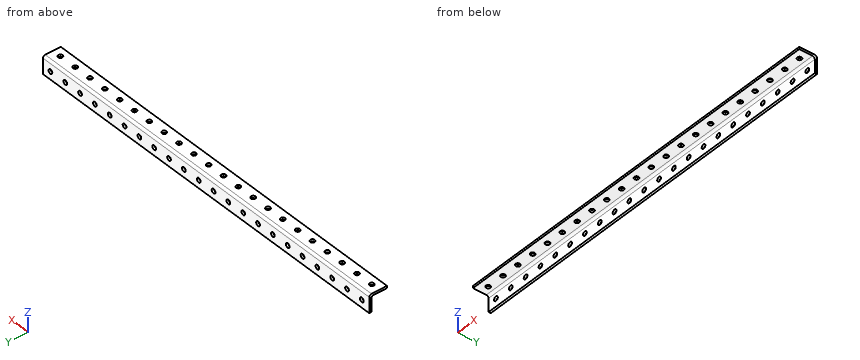
Autodesk Inventor part; units mm, degrees
ref_plane "YZ Plane" through (0, 0, 0) normal (1, 0, 0) x (0, 1, 0)
ref_plane "XZ Plane" through (0, 0, 0) normal (0, 1, 0) x (-1, 0, 0)
ref_plane "XY Plane" through (0, 0, 0) normal (0, 0, 1) x (1, 0, 0)
sketch "Sketch1" plane through (0, 0, 0) normal (1, 0, 0) x (0, 1, 0)
  line L0 (0, 0) -> (22.225, 0)
  line L1 (25.4, -3.175) -> (25.4, -25.4)
  line L2 (22.2268, -25.4) -> (22.2268, -6.3482)
  line L3 (19.0518, -3.1732) -> (0, -3.1732)
  line L4 (25.4, -25.4) -> (22.2268, -25.4)
  line L5 (0, 0) -> (0, -3.1732)
  arc A0 (25.4, -3.175) -> (22.225, 0) centre (22.225, -3.175) ccw
  arc A1 (22.2268, -6.3482) -> (19.0518, -3.1732) centre (19.0518, -6.3482) ccw
  point P0 (25.4, 0)
  dimension "d0" = 25.4
  dimension "d1" = 25.4
  dimension "d2" = 3.175
extrude "Extrusion1" add sketch "Sketch1" along normal blind 558.8
sketch "Sketch2" plane through (0, 0, 0) normal (0, 0, 1) x (1, 0, 0)
  line L0 (0, 0) -> (0, 22.225)
  circle A0 centre (12.7, 11.1125) radius 1.9225
  dimension "d5" = 12.7
hole "Hole1" at (12.7, 11.1125, 0) direction (0, 0, -1) diameter 6.35 end through all
pattern_linear "Rectangular Pattern1" count 24 spacing 25.4 along (1, 0, 0) of "Hole1"
sketch "Sketch3" plane through (0, 25.4, -3.175) normal (0, 1, 0) x (1, 0, 0)
  line L0 (0, 0) -> (0, 22.225)
  circle A0 centre (12.7, 11.1125) radius 5.2364
  point P0 (0, -3.175)
  dimension "d16" = 12.7
hole "Hole2" at (12.7, 25.4, -14.2875) direction (0, -1, 0) diameter 6.35 end through all
pattern_linear "Rectangular Pattern2" count 24 spacing 25.4 along (1, 0, 0) of "Hole2"
properties part number "frame_angle_horiz" material "Steel, Mild"
Input: part model. Units: mm. Frame: model coordinates. Round coordinates to 2 decimals unless told otherwise and drop trailing zeros. Loops run counter-clockwise (first coordinate to the right, second up) from the corner with the lowest first, then second, coordinate; pieces in that order, holes last. Notation, with made-up numbers: (83.5, 75.5) -> (97.5, 75.5) arc R10 cw to (97.5, 84.5) -> close; hole circle Ø2 at (77.5, 65.5). An arc over 180 degrees is marked (long way). Use one line per item in the form item = value. Start each with the question number.
Item 1: Material intervals for L1, parallel to Z at x = 396.5, y = 7.5; L2, parallel to Y at x = 429, z = -6.5; L3, parallel to Y at x = 266.7, z = -2.5, sorted ascending. Write a range as from..to.
Item 2: Section query A-A on x = 434.5. Return the cut outline in (y, z) (3 decimals), then the cut area to 3 significant figures.
Item 3: Contact query for flat-ended pins moving along their axis: pin 1 Ø4 at (x, y) = (469.9, 11.11) entering from -Z; pin 2 Ø12 at (x, y) = (130.5, 7) entering from -Z; pin 3 Ø8.5 at (x, z) = (520.7, -14.29) entering from -Y. Output: stop coordinate, or through.
Ans:
q1.L1 = -3.17..0
q1.L2 = 22.23..25.4
q1.L3 = 0..7.94, 14.29..25.33
q2.outline = (0, -3.173) -> (19.052, -3.173) arc R3.175 cw to (22.227, -6.348) -> (22.227, -25.4) -> (25.4, -25.4) -> (25.4, -3.175) arc R3.175 ccw to (22.225, 0) -> (0, 0) -> close
q2.area = 151 mm^2
q3.pin_1 = through
q3.pin_2 = -3.17
q3.pin_3 = 22.23
